Verification items for the finished model (mm, model axes). Round coordinates to 2 decimals unless told otherwise and drop trailing zeros. Write each loop counter-clockwise with the first axis right and the second up, starting at its lowest first coordinate (ties: lowest second). Pieces come first, ordered by that corner, then holes. Notation, with made-up numbers: (9, 85) -> (34, 85) arc R14 cw to (34, 96) -> close; hole circle Ø4 at (7.5, -25.5). An arc over 180 degrees is marked (long way). Answer as a JSON object with one key per item and string values. Group by question number.
(1) Sectioned sample at C-C on x = 13. Record the cut outline in (y, z), and give its area (3 significant figures).
(2) Sectioned sample at A-A on z = 2.5. Record the cut outline in (x, y) (3 decimals), and give its area (3 significant figures).
(3) Sectioned sample at B-B on x = 0. Record the cut outline in (y, z) (3 decimals), and give its area (3 significant figures).
(4) Draft check along Y on faces 1 (the face through (-13.81, -7.82, 9.52)), 2 (the face through (14.354, 8.133, 4.383)), 3 (the face through (12, 3, 10.16)), 4 (the face through (-7.559, 5.796, 4.079)). Enter one of: released by +Y, released by -Y, zero draft, split by the parting line, or undercut.
(5) Scan lines: L1, parallel to Y at x = 0, z = 3.5 (3 decimals); L2, parallel to X at y = 0.5, z = 9; L3, parallel to X at y = 4, z = 7.5. Record each from-to range of solid material in increasing order. Write a range as from..to.
(6) Sectioned sample at D-D on y = 14.5. Record the cut outline in (x, z).
(7) Gauge pin test, flat ends, axial feed: pin 1 Ø6 at (x, y) = (-2, 8) entering from +Z; pin 2 Ø4 at (y, z) = (9.5, 4.5) entering from -X; pin 3 Ø3 at (y, z) = (-8.5, 7) entering from +X. Record the tip position at first contact, or that the pin passes through.
Solid Edge part; units mm, degrees
sketch "Sketch1" plane through (0, 0, 0) normal (0, 0, 1) x (1, 0, 0)
  line L0 (-19.05, 0) -> (-9.525, -16.4978)
  line L1 (-9.525, -16.4978) -> (9.525, -16.4978)
  line L2 (9.525, -16.4978) -> (19.05, 0)
  line L3 (19.05, 0) -> (9.525, 16.4978)
  line L4 (9.525, 16.4978) -> (-9.525, 16.4978)
  line L5 (-9.525, 16.4978) -> (-19.05, 0)
  circle A0 centre (0, 0) radius 9.525
extrude "Protrusion1" add sketch "Sketch1" along normal blind 10.16
fillet "Round_1" radius 2.54 1 edges at (-9.525, 0, 10.16)
fillet "Round1" radius 0.635 1 edges at (-9.525, 0, 0)
chamfer "Chamfer_3" distance 1.27 angle 45 6 edges at (14.2875, 8.2489, 10.16) (14.2875, -8.2489, 10.16) (0, -16.4978, 10.16) (-14.2875, -8.2489, 10.16) (-14.2875, 8.2489, 10.16) (0, 16.4978, 10.16)
Computed values:
{
 "1": {"outline": "(-10.48, 0) -> (10.48, 0) -> (10.48, 8.89) -> (7.94, 10.16) -> (-7.94, 10.16) -> (-10.48, 8.89) -> close", "area": "210 mm2"},
 "2": {"outline": "(-19.05, 0) -> (-9.525, -16.498) -> (9.525, -16.498) -> (19.05, 0) -> (9.525, 16.498) -> (-9.525, 16.498) -> close; hole circle Ø19.05 at (0, 0)", "area": "658 mm2"},
 "3": {"outline": "(-16.498, 0) -> (-10.16, 0) arc R0.635 ccw to (-9.525, 0.635) -> (-9.525, 7.62) arc R2.54 ccw to (-12.065, 10.16) -> (-15.228, 10.16) -> (-16.498, 8.89) -> close; (9.525, 0.635) arc R0.635 ccw to (10.16, 0) -> (16.498, 0) -> (16.498, 8.89) -> (15.228, 10.16) -> (12.065, 10.16) arc R2.54 ccw to (9.525, 7.62) -> close", "area": "137 mm2"},
 "4": {"face 1": "released by -Y", "face 2": "released by +Y", "face 3": "zero draft", "face 4": "undercut"},
 "5": {"L1": "-16.498..-9.525, 9.525..16.498", "L2": "-18.63..-9.92, 9.92..18.63", "L3": "-16.74..-8.64, 8.64..16.74"},
 "6": {"outline": "(-10.68, 0) -> (10.68, 0) -> (10.68, 8.89) -> (9.21, 10.16) -> (-9.21, 10.16) -> (-10.68, 8.89) -> close"},
 "7": {"pin 1": "z = 10.02", "pin 2": "x = -14.72", "pin 3": "x = 15.01"}
}
